For this review, take the finished solid that the model builds, in its own axes (mm). Face numbers are marked on the shaded views. A direction names the side the tool comes from. Give positions to 0.01 mm unless a question says otherwise; leave off trailing zeros. Loops run counter-clockwise (first coordinate to the right, second up) from the corner with the lowest first, then second, coordinate; pieces in that order, holes last.
```python
from build123d import *

# Parameters (mm, degrees)
BASE_R              = 40
BOSS_EXTRUDE1_DEPTH = 10
STOPPER_R           = 20.75
BOSS_EXTRUDE2_DEPTH = 20
FILLET1_R           = 10


with BuildPart() as part:
    # base → Boss-Extrude1 (new body)
    with BuildSketch(Plane(origin=(0, 0, 0), x_dir=(1, 0, 0), z_dir=(0, 1, 0))):
        with Locations(Location((0, 0, 0), (0, 0, 270))):
            Circle(BASE_R)
    extrude(amount=-BOSS_EXTRUDE1_DEPTH)

    # stopper → Boss-Extrude2 (add)
    with BuildSketch(Plane(origin=(0, 0, 0), x_dir=(1, 0, 0), z_dir=(0, 1, 0))):
        with Locations(Location((0, 0, 0), (0, 0, 270))):
            Circle(STOPPER_R)
    extrude(amount=BOSS_EXTRUDE2_DEPTH)

    # Fillet1
    fillet1_edges = [part.edges().sort_by_distance(p)[0] for p in [
        (0, -10, -40),
    ]]
    fillet(fillet1_edges, radius=FILLET1_R - 0.0001)  # a hair under: the kernel refuses the full size


solid = part.part
```
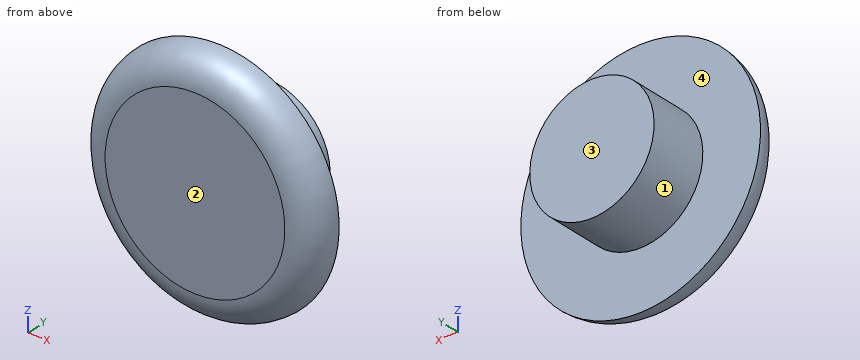
Q1. Consider section C-C on y = 1.25. Give the boundary of the cut face in (x, z).
Answers:
outline: circle Ø41.5 at (0, 0)
Q2. For probe 1 along Y at (x, z) = (-4.5, 26.5); probe 2 along X at (y, z) = (2.25, 0); probe 3 along X at (y, z) = (-0.5, -6.5), list the stretches that pass through material, from the lowest coordinate up.
Answers:
probe 1: y = -10 to 0
probe 2: x = -20.75 to 20.75
probe 3: x = -39.46 to 39.46
Q3. For pin 1 Ø4 at (x, y) = (-8.5, -3) entering from -Z; pin 2 Ø10 at (x, z) = (17, -12) entering from +Y; pin 3 Ø3 at (y, z) = (-4.5, -29.5) entering from +X; pin 4 Ø5 at (x, y) = (8, -3.5) entering from +Z, all flat-tipped, find the tip position at first contact; note any pin that passes through.
Answers:
pin 1: stops at z = -39.24
pin 2: stops at y = 20
pin 3: stops at x = 27.33
pin 4: stops at z = 39.36
Q4. Machinability: for the marked faces 3 and 4, which of the approach directions +Z, -Z, +X, -X, +Y, -Y give a long, thin tool a straight path to every point of the face, cutting with its end or side? Answer none if there is none.
Answers:
face 3: +Z, -Z, +X, -X, +Y
face 4: +Y
Q5. Mouldability with a two-part tool opening along Z and no side actions: class the marked faces 1 and 2 as +Z half, -Z half, draft (parallel to the pull), parting line (faces both ways), or undercut.
Answers:
face 1: parting line
face 2: draft
